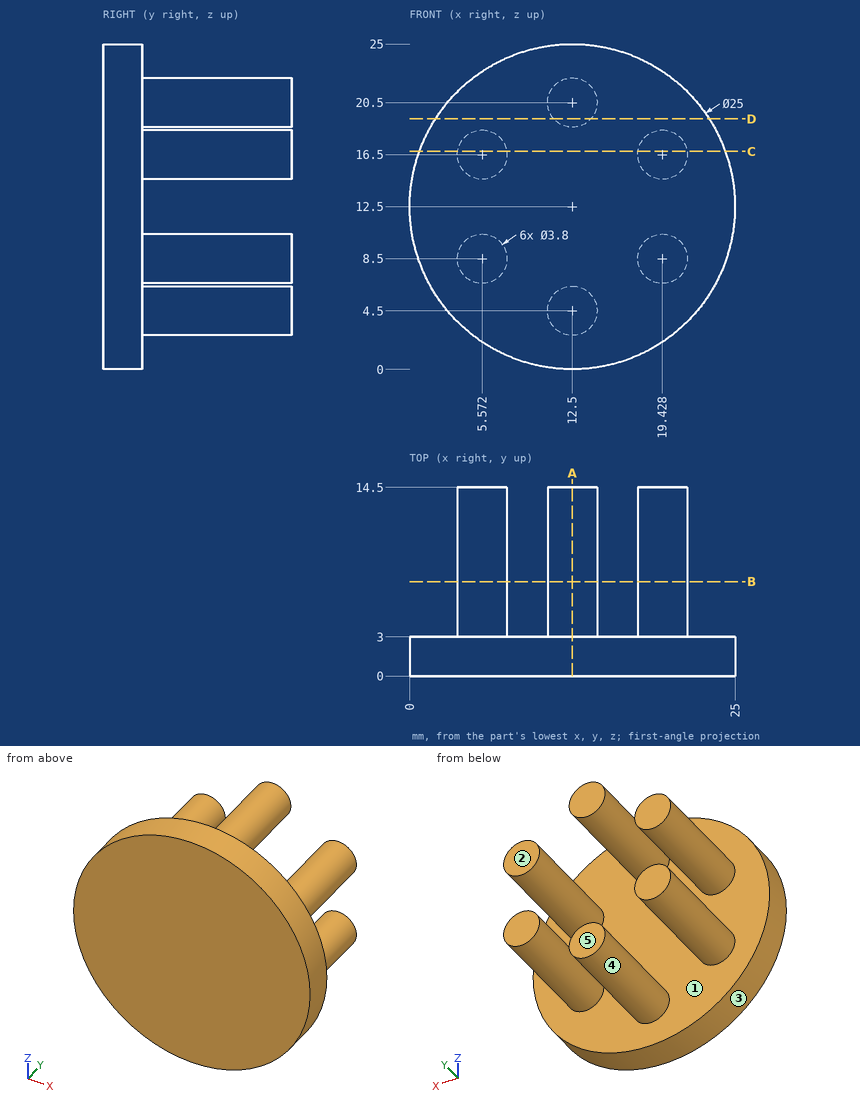
Job drawing, mm, ordinate dimensions from the low corner. One solid piece. A direction names the side the tool comes from. Round coordinates to 2 decimals unless told otherwise and drop trailing zeros. Loops run counter-clockwise (first coordinate to the right, second up) from the corner with the lowest first, then second, coordinate; pieces in that order, holes last.
(1) Two-plate mould, pull along Z, no slides. Class the marked faces 1, 2 and 3: +Z half, -Z half, draft (parallel to the pull), parting line (faces both ways), or undercut.
(2) Cut at D-D (z = 19.25). Give the cut face in (x, y).
(3) Wall check: line 1 along Y through (x, z) = (2.5, 10.75); line 2 along X through (y, z) = (10.5, 16.25) (1 decimal); line 3 along Z through (x, y) = (19, 12.25). Give the ranges that are in metal, low to high.
(4) Drop flat-ended pins along their axis: pin 1 (3 mm diameter, centred on x = 14.5, y = 12, fed in from +Z); pin 2 (1.5 mm diameter, centred on x = 13, z = 16, fed in from -Y); pin 3 (8 mm diameter, centred on x = 6, y = 9.5, fed in from -Z); pin 4 (2 mm diameter, centred on x = 5.5, y = 3.5, fed in from -Z). Give the stop position or say it passes through.
(5) Which spindle directions (+Z, -Z, +X, -X, +Y, -Y) get a long thin tool onto all of the face, cutting with end or side? Do the marked faces 4 and 5. Say none if no direction does.
(6) Cut at C-C (z = 16.75). Give the cut face in (x, y) (1 decimal).
(7) Cut at A-A (x = 12.5). Give the cut face in (y, z), plus the area to 3 significant figures.
(8) Cut at B-B (y = 7.25). Give the cut face in (x, z).
Findings below:
1. face 1: undercut
1. face 2: draft
1. face 3: parting line
2. outline: (1.98, 0) - (23.02, 0) - (23.02, 3) - (13.93, 3) - (13.93, 14.5) - (11.07, 14.5) - (11.07, 3) - (1.98, 3) - close
3. line 1: y = 0 to 3
3. line 2: x = 3.7 to 7.5, 17.5 to 21.3
3. line 3: z = 6.65 to 10.35, 14.65 to 18.35
4. pin 1: stops at z = 22.33
4. pin 2: stops at y = 0
4. pin 3: stops at z = 6.6
4. pin 4: stops at z = 1.61
5. face 4: +Y
5. face 5: +Z, -Z, +X, -X, +Y
6. outline: (0.7, 0) - (24.3, 0) - (24.3, 3) - (21.3, 3) - (21.3, 14.5) - (17.5, 14.5) - (17.5, 3) - (7.5, 3) - (7.5, 14.5) - (3.7, 14.5) - (3.7, 3) - (0.7, 3) - close
7. outline: (0, 0) - (3, 0) - (3, 2.6) - (14.5, 2.6) - (14.5, 6.4) - (3, 6.4) - (3, 18.6) - (14.5, 18.6) - (14.5, 22.4) - (3, 22.4) - (3, 25) - (0, 25) - close
7. area: 162 mm2
8. outline: circle Ø3.8 at (5.57, 8.5); circle Ø3.8 at (5.57, 16.5); circle Ø3.8 at (12.5, 4.5); circle Ø3.8 at (12.5, 20.5); circle Ø3.8 at (19.43, 8.5); circle Ø3.8 at (19.43, 16.5)
